from build123d import *

# Parameters (mm, degrees)
SKETCH_1_W          = 510
SKETCH_1_H          = 20
SKETCH_1_R          = 5
SKETCH_1_W_2        = 20
SKETCH_1_H_2        = 410
EXTRUDE_1_DEPTH     = 20
SKETCH_2_R          = 5
CUT_EXTRUDE_1_DEPTH = 20


with BuildPart() as part:
    # Эскиз1 → Бобышка-Вытянуть1 (new body)
    # profile 1 of 3: a face of its own
    with BuildSketch(Plane.XY):
        with Locations((-10, 0)):
            Rectangle(SKETCH_1_W, SKETCH_1_H)
        with Locations((-245, 0)):
            Circle(SKETCH_1_R, mode=Mode.SUBTRACT)
    # profile 2 of 3: a face of its own
    with BuildSketch(Plane.XY):
        with Locations((255, 0)):
            Rectangle(SKETCH_1_W_2, SKETCH_1_H)
    # profile 3 of 3: a face of its own
    with BuildSketch(Plane.XY):
        with Locations((255, -215)):
            Rectangle(SKETCH_1_W_2, SKETCH_1_H_2)
    extrude(amount=EXTRUDE_1_DEPTH)

    # Эскиз2 → Вырез-Вытянуть1 (cut)
    with BuildSketch(Plane.XY.offset(20)):
        with Locations((255, -400)):
            Circle(SKETCH_2_R)
    extrude(amount=-CUT_EXTRUDE_1_DEPTH, mode=Mode.SUBTRACT)


solid = part.part
The listing builds one solid part. Answer for the finished solid, in the listing's coordinates (mm). A direction names the side the tool comes from. Give positions to 0.01 mm unless a question says otherwise; leave off trailing zeros. Loops run counter-clockwise (first coordinate to the right, second up) from the corner with the lowest first, then second, coordinate; pieces in that order, holes last.
Item 1: A tool of negligible diameter and unlimited length cuts with its end or side. For faces 1 (the flat face through (245, -218, 10)), 2 (the flat face through (117, 3, 0)), from which of +Z, -Z, +X, -X, +Y, -Y can it reach the whole face along a straight path? Write none if from no direction.
Derived:
face 1: +Z, -Z, -X, -Y
face 2: -Z, +X, -X, +Y, -Y
Item 2: A cutting plane is placed at C-C (x = 166.5). Give the vertices of the cut face in (y, z), then the cut area to 3 significant figures.
Derived:
outline: (-10, 0) - (10, 0) - (10, 20) - (-10, 20) - close
area: 400 mm2
Item 3: A cutting plane is placed at A-A (z = 5). Give the vertices of the cut face in (x, y), then the cut area to 3 significant figures.
Derived:
outline: (-265, -10) - (245, -10) - (245, -420) - (265, -420) - (265, 10) - (-265, 10) - close; hole circle Ø10 at (-245, 0); hole circle Ø10 at (255, -400)
area: 18,600 mm2
Item 4: Each of these flat-tipped pins is pushed along its axis until it touches: pin 1 Ø3 at (x, z) = (-99.5, 16.5) entering from -Y; pin 2 Ø5 at (y, z) = (-280.5, 13.5) entering from -X. Where does it stop, or does it pass through?
Derived:
pin 1: stops at y = -10
pin 2: stops at x = 245
Item 5: Find the intervals of material crossed by line 1 along Y through (x, z) = (255, 6.5); line 2 along X through (y, z) = (-400, 12.5); line 3 along Y through (x, z) = (-245, 5.5), in increasing order.
Derived:
line 1: y = -420 to -405, -395 to 10
line 2: x = 245 to 250, 260 to 265
line 3: y = -10 to -5, 5 to 10
Item 6: A cutting plane is placed at B-B (y = -362). Give the vertices of the cut face in (x, z).
Derived:
outline: (245, 0) - (265, 0) - (265, 20) - (245, 20) - close
